Work out the finished part from the listing and answer in its coordinate system (mm). A direction names the side the tool comes from. Coordinates: 2 decimals unless noted, no trailing zeros. Order: outer loops, then holes, each group sorted by start corner. A loop starts at its lowest first (then second) coordinate and runs counter-clockwise, first axis right, second up. Notation, with made-up numbers: (-17.75, -12) -> (-3.75, -12) arc R34 cw to (-3.75, 22) -> close; hole circle Ø10 at (-1, 72.5). An arc over 180 degrees is marked (long way). Write item = value, one per line. Start each with the question number.
Q1. Straight lines are drawn through the part: L1, parallel to X at y = -6, z = -17.5; L2, parallel to Z at x = -12.11, y = -5.9; L3, parallel to Z at x = -12, y = 1.25. For each, find the intervals that lie inside material, in ascending order. Write a range as from..to.
Q2. Which of the six approach directions +Z, -Z, +X, -X, +Y, -Y give full straight-line access (tool end or side, diameter ignored) to faces 4 (the flat face through (39.31, -5, -19)), 5 (the cylindrical face through (20.03, 0.89, -21.37)), 6 (the flat face through (-14, -4, -2)), 7 (the flat face through (37.33, -8.02, 3.86))?
Q3. The part is cut by section B-B, the plane x = 0. Count the separate pieces of the cut face and the enclosed holes in it, plus the area to 3 significant figures.
Q4. The part is cut by section A-A, the plane z = -10.25. Determine the outline of the cut face in (x, y).
Q5. The part is cut by section C-C, the plane x = 29. Determine the outline of the cut face in (y, z), plus the area to 3 significant figures.
Q6. For a pull along Z with two mould halves and no side action, classify faces 1 (the flat face through (7, 1, -3)), 2 (the flat face through (-4.4, -8.09, -24.36)), 3 (the flat face through (4, -3, -25.5)) as +Z half, -Z half, draft (parallel to the pull), parting line (faces both ways), or undercut.
Q7. Flat-ended cylindrical pins translate along their axes: pin 1 (2.5 mm diameter, centred on x = -12.11, z = -3, fed in from -Y); pin 2 (6 mm diameter, centred on x = -12.11, z = -3, fed in from +Y); pin 3 (3 mm diameter, centred on x = 20.7, z = 0, fed in from +Y); pin 4 (3 mm diameter, centred on x = 20.7, z = -20.5, fed in from -Y). Find the tip coordinate at first contact, or state that the pin passes through.
```python
from build123d import *

# Parameters (mm, degrees)
ESQUISSE1_W                                        = 53.8
ESQUISSE1_H                                        = 26.5
ESQUISSE1_R                                        = 1.1
BOSS_EXTRU_1_DEPTH                                 = 3
CHAMBRAGE_POUR_VIS_SIX_PANS_CREUX_M1_6_D           = 2.2
CHAMBRAGE_POUR_VIS_SIX_PANS_CREUX_M1_6_CBORE_D     = 3.8
CHAMBRAGE_POUR_VIS_SIX_PANS_CREUX_M1_6_CBORE_DEPTH = 1.2
BOSS_EXTRU_2_START                                 = 16
BOSS_EXTRU_2_DEPTH                                 = 19
ESQUISSE6_W                                        = 11.6
ESQUISSE6_H                                        = 6
ENL_V_MAT_EXTRU_1_DEPTH                            = 60.582531836
ENL_V_MAT_EXTRU_2_DEPTH                            = 58.559344159
ENL_V_MAT_EXTRU_2_DEPTH_BACK                       = 58.559344159
ESQUISSE7_R                                        = 1.6
PER_AGEAVANC_1_START                               = -4
PER_AGEAVANC_1_OUTLINE_R                           = 3.25
PER_AGEAVANC_1_OUTLINE_R_2                         = 1.6
PER_AGEAVANC_1_DEPTH                               = 7
BOSS_EXTRU_3_DEPTH                                 = 2
ESQUISSE11_R                                       = 3.860993261
BOSS_EXTRU_4_DEPTH                                 = 13
ESQUISSE12_W                                       = 8
ESQUISSE12_H                                       = 30.5
ENL_V_MAT_EXTRU_3_DEPTH                            = 59.404435619
CHANFREIN1_SIZE                                    = 1
CONG_1_R                                           = 5
CHANFREIN2_SIZE                                    = 2


with BuildPart() as part:
    # Esquisse1 → Boss.-Extru.1 (new body)
    with BuildSketch(Plane(origin=(0, 0, 0), x_dir=(1, 0, 0), z_dir=(0, 1, 0))):
        with Locations((16.5, 10.25)):
            Rectangle(ESQUISSE1_W, ESQUISSE1_H)
        with Locations(Location((0, 0, 0), (0, 0, 270))):
            Circle(ESQUISSE1_R, mode=Mode.SUBTRACT)
        with Locations(Location((20.7, 0, 0), (0, 0, 270))):
            Circle(ESQUISSE1_R, mode=Mode.SUBTRACT)
        with Locations(Location((0, 20.5, 0), (0, 0, 270))):
            Circle(ESQUISSE1_R, mode=Mode.SUBTRACT)
        with BuildLine():
            Line((-5.4, 3), (-5.4, 17.5))
            Line((-5.4, 17.5), (19.829743733, 17.5))
            ThreePointArc((19.829743733, 17.5), (32.837694897, 21.29211021), (40.69, 10.25))
            ThreePointArc((40.69, 10.25), (32.837694897, -0.79211021), (19.829743733, 3))
            Line((19.829743733, 3), (-5.4, 3))
        make_face(mode=Mode.SUBTRACT)
        with Locations(Location((20.7, 20.5, 0), (0, 0, 270))):
            Circle(ESQUISSE1_R, mode=Mode.SUBTRACT)
    extrude(amount=BOSS_EXTRU_1_DEPTH)

    # Chambrage pour vis à six pans creux M1.61 (through all)
    with Locations(Plane(origin=(0, 3, 0), x_dir=(1, 0, 0), z_dir=(0, 1, 0))):
        with Locations((0, 20.5), (20.7, 20.5), (20.7, 0), (0, 0)):
            CounterBoreHole(CHAMBRAGE_POUR_VIS_SIX_PANS_CREUX_M1_6_D / 2, CHAMBRAGE_POUR_VIS_SIX_PANS_CREUX_M1_6_CBORE_D / 2, CHAMBRAGE_POUR_VIS_SIX_PANS_CREUX_M1_6_CBORE_DEPTH)

    # Esquisse4 → Boss.-Extru.2 (add)
    with BuildSketch(Plane.XZ.offset(BOSS_EXTRU_2_START)):
        Polygon((-10.4, 3), (-17.91, 3), (-17.91, -23.5), (-10.4, -23.5), (-6.31, -23.5), (-6.31, 3), align=None)
        with BuildLine():
            Line((39.31, 3), (50.91, 3))
            Line((50.91, 3), (50.91, -23.5))
            Line((50.91, -23.5), (39.31, -23.5))
            Line((39.31, -23.5), (39.31, -15.759990926))
            ThreePointArc((39.31, -15.759990926), (40.69, -10.25), (39.31, -4.740009074))
            Line((39.31, -4.740009074), (39.31, 3))
        make_face()
    extrude(amount=-BOSS_EXTRU_2_DEPTH)

    # Esquisse6 → Enlèv. mat.-Extru.1 (cut, through all)
    with BuildSketch(Plane(origin=(0, 0, -23.5), x_dir=(-1, 0, 0), z_dir=(0, 0, -1))):
        with Locations((12.11, -13)):
            Rectangle(ESQUISSE6_W, ESQUISSE6_H)
        with Locations((-45.11, -13)):
            Rectangle(ESQUISSE6_W, ESQUISSE6_H)
    extrude(amount=-ENL_V_MAT_EXTRU_1_DEPTH, mode=Mode.SUBTRACT)

    # Esquisse7 → Enlèv. mat.-Extru.2 (cut, two sides: drawn at the far end of the back side and taken through both)
    with BuildSketch(Plane.XZ.offset(10).offset(-ENL_V_MAT_EXTRU_2_DEPTH_BACK)):
        with Locations(Location((-12.11, -3, 0), (0, 0, 270))):
            Circle(ESQUISSE7_R)
        with Locations(Location((-12.11, -17.5, 0), (0, 0, 270))):
            Circle(ESQUISSE7_R)
        with Locations(Location((45.11, -10.25, 0), (0, 0, 270))):
            Circle(ESQUISSE7_R)
    extrude(amount=ENL_V_MAT_EXTRU_2_DEPTH + ENL_V_MAT_EXTRU_2_DEPTH_BACK, mode=Mode.SUBTRACT)

    # PerçageAvancé1: read off the stored shape, not the designer's step
    # PerçageAvancé1 outline → PerçageAvancé1 (cut)
    # profile 1 of 3: a face of its own
    with BuildSketch(Plane(origin=(0, 0, 0), x_dir=(1, 0, 0), z_dir=(0, 1, 0)).offset(PER_AGEAVANC_1_START)):
        with Locations((-12.11, 17.5)):
            Circle(PER_AGEAVANC_1_OUTLINE_R)
        with Locations((-12.11, 17.5)):
            Circle(PER_AGEAVANC_1_OUTLINE_R_2, mode=Mode.SUBTRACT)
    # profile 2 of 3: a face of its own
    with BuildSketch(Plane(origin=(0, 0, 0), x_dir=(1, 0, 0), z_dir=(0, 1, 0)).offset(PER_AGEAVANC_1_START)):
        with Locations((-12.11, 3)):
            Circle(PER_AGEAVANC_1_OUTLINE_R)
        with Locations((-12.11, 3)):
            Circle(PER_AGEAVANC_1_OUTLINE_R_2, mode=Mode.SUBTRACT)
    # profile 3 of 3: a face of its own
    with BuildSketch(Plane(origin=(0, 0, 0), x_dir=(1, 0, 0), z_dir=(0, 1, 0)).offset(PER_AGEAVANC_1_START)):
        with Locations((45.11, 10.25)):
            Circle(PER_AGEAVANC_1_OUTLINE_R)
        with Locations((45.11, 10.25)):
            Circle(PER_AGEAVANC_1_OUTLINE_R_2, mode=Mode.SUBTRACT)
    extrude(amount=PER_AGEAVANC_1_DEPTH, mode=Mode.SUBTRACT)

    # Esquisse10 → Boss.-Extru.3 (add)
    with BuildSketch(Plane.XY.offset(3)):
        Polygon((-6.31, -10), (-1.31, -5), (34.31, -5), (39.31, -10), (50.91, -10), (50.91, 3), (-17.91, 3), (-17.91, -10), align=None)
    boss_extru_3 = extrude(amount=BOSS_EXTRU_3_DEPTH)

    # Symétrie1: Boss.-Extru.3 across plane
    add(boss_extru_3.mirror(Plane.XY.offset(-10.25)))

    # Esquisse11 → Boss.-Extru.4 (add)
    with BuildSketch(Plane(origin=(0, 3, 0), x_dir=(1, 0, 0), z_dir=(0, 1, 0))):
        with Locations((45.11, 10.25)):
            Circle(ESQUISSE11_R)
    extrude(amount=-BOSS_EXTRU_4_DEPTH)

    # Esquisse12 → Enlèv. mat.-Extru.3 (cut, through all)
    with BuildSketch(Plane(origin=(0, 3, 0), x_dir=(1, 0, 0), z_dir=(0, 1, 0))):
        with Locations((46.91, 10.25)):
            Rectangle(ESQUISSE12_W, ESQUISSE12_H)
    extrude(amount=-ENL_V_MAT_EXTRU_3_DEPTH, mode=Mode.SUBTRACT)

    # Chanfrein1
    chanfrein1_edges = [part.edges().sort_by_distance(p)[0] for p in [
        (-17.91, -3.5, 5),
        (-17.91, -3.5, -25.5),
        (12.5, 3, -25.5),
        (12.5, 3, 5),
        (-17.91, 3, -10.25),
    ]]
    chamfer(chanfrein1_edges, length=CHANFREIN1_SIZE)

    # Congé1
    cong_1_edges = [part.edges().sort_by_distance(p)[0] for p in [
        (42.91, -4, -25.5),
        (42.91, -4, 5),
    ]]
    fillet(cong_1_edges, radius=CONG_1_R)

    # Chanfrein2
    chanfrein2_edges = [part.edges().sort_by_distance(p)[0] for p in [
        (-6.31, -5, -23.5),
        (-6.31, -5, 3),
        (39.31, -5, 3),
        (39.31, -5, -23.5),
    ]]
    chamfer(chanfrein2_edges, length=CHANFREIN2_SIZE)


solid = part.part
```
Model answer:
q1.L1 = -17.91..-13.71, -10.51..-6.31, 39.31..42.91
q1.L2 = -25.5..-19.1, -15.9..-4.6, -1.4..5
q1.L3 = -25.5..-20.75, -14.25..-6.25, 0.25..5
q2.face_4 = -Y
q2.face_5 = +Y, -Y
q2.face_6 = +Y
q2.face_7 = +Z, -Z, -Y
q3.separate_pieces = 4
q3.enclosed_holes = 0
q3.area = 50.0 mm2
q4.outline = (-17.91, -10) -> (-6.31, -10) -> (-6.31, 0) -> (-5.4, 0) -> (-5.4, 3) -> (-16.91, 3) -> (-17.91, 2) -> close; (40.69, -10) -> (42.91, -10) -> (42.91, 3) -> (40.69, 3) -> close
q5.outline = (-5, -25.5) -> (2, -25.5) -> (3, -24.5) -> (3, -21.94) -> (0, -21.94) -> (0, -23.5) -> (-5, -23.5) -> close; (-5, 3) -> (0, 3) -> (0, 1.44) -> (3, 1.44) -> (3, 4) -> (2, 5) -> (-5, 5) -> close
q5.area = 40.4 mm2
q6.face_1 = undercut
q6.face_2 = draft
q6.face_3 = -Z half
q7.pin_1 = through
q7.pin_2 = -4
q7.pin_3 = 1.8
q7.pin_4 = 0
